Job drawing, mm, ordinate dimensions from the low corner. One solid piece. A direction names the side the tool comes from. Round coordinates to 2 decimals unless told otherwise and drop trailing zeros. Loops run counter-clockwise (first coordinate to the right, second up) from the corner with the lowest first, then second, coordinate; pieces in that order, holes last.
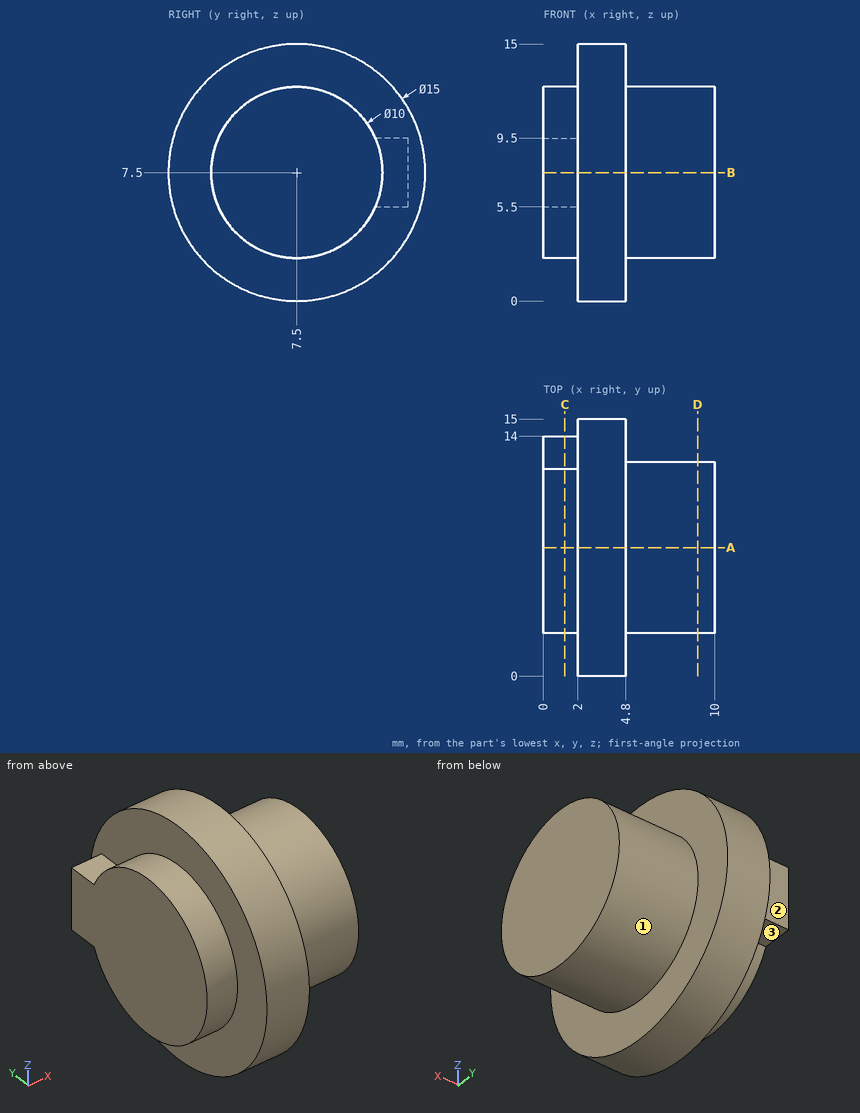
(1) Slice it at D-D on x = 9. List the corners of the cut face in (y, z), plus the area to 3 significant figures.
Responses:
outline: circle Ø10 at (7.5, 7.5)
area: 78.5 mm2
(2) Which spindle directions (+Z, -Z, +X, -X, +Y, -Y) get a long thin tool onto all of the face, cutting with end or side? Do the marked faces 1, 2 and 3. Say none if no direction does.
Responses:
face 1: +X
face 2: +Z, -Z, -X, +Y
face 3: -Z, -X, +Y
(3) Slice it at C-C on x = 1.25. List the corners of the cut face in (y, z), plus the area to 3 significant figures.
Responses:
outline: (12.08, 5.5) - (14, 5.5) - (14, 9.5) - (12.08, 9.5) arc R5 ccw (long way) to start
area: 85.1 mm2
(4) Pin check, flat tips, straight feed: P1, Ø0.6, axis at x = 1, y = 13, coming from the +Z side; P2, Ø1, axis at x = 3, y = 3, coming from the -Z side; P3, Ø6, axis at x = 7.5, z = 8, coming from the +Y side; P4, Ø3, axis at x = 6, z = 12, coming from the -Y side. Stop position of each tip, or through.
Responses:
P1: stops at z = 9.5
P2: stops at z = 1.16
P3: stops at y = 15
P4: stops at y = 0.92
(5) Slice it at A-A on y = 7.5. List the corners of the cut face in (x, z).
Responses:
outline: (0, 2.5) - (2, 2.5) - (2, 0) - (4.8, 0) - (4.8, 2.5) - (10, 2.5) - (10, 12.5) - (4.8, 12.5) - (4.8, 15) - (2, 15) - (2, 12.5) - (0, 12.5) - close
(6) Probe line 1 (X direction, y = 3.75, z = 1.25); line 2 (Z direction, x = 1.25, y = 10.5); line 3 (Y direction, x = 6.25, z = 11). List the from-to ranges inside material, lowest first.
Responses:
line 1: x = 2 to 4.8
line 2: z = 3.5 to 11.5
line 3: y = 3.93 to 11.07
(7) Slice it at B-B on z = 7.5. List the corners of the cut face in (x, y).
Responses:
outline: (0, 2.5) - (2, 2.5) - (2, 0) - (4.8, 0) - (4.8, 2.5) - (10, 2.5) - (10, 12.5) - (4.8, 12.5) - (4.8, 15) - (2, 15) - (2, 14) - (0, 14) - close
